Work out the finished part from the listing and answer in its coordinate system (mm). A direction names the side the tool comes from. Give positions to 0.01 mm unless a question says otherwise; leave off trailing zeros. Loops run counter-clockwise (first coordinate to the right, second up) from the corner with the lowest first, then second, coordinate; pieces in that order, holes last. Notation, with made-up numbers: M 48,-18.75 L 98,-18.75 A29 ccw 98,1.25 Z; hole C 17.5,-33 d2. An arc over 180 degrees is marked long. Use a Markdown table: item, result.
```python
from build123d import *

# Parameters (mm, degrees)
F1_DEPTH      = 10
F3_W          = 3
F3_H          = 10
F4_DEPTH      = 9.464
F5_W          = 7
F5_H          = 14
F5_W_2        = 3
F5_H_2        = 10
F6_DEPTH      = 3
F6_DEPTH_BACK = 1
F7_R          = 0.5


with BuildPart() as f1:
    # F0 (on Top) → F1 (new body)
    with BuildSketch(Plane.XY):
        Polygon((-13.856406, 0), (0, 0), (-3.464102, 6), align=None)
    extrude(amount=F1_DEPTH)

    # F3 (on offset) → F4 (join)
    with BuildSketch(Plane.YZ.offset(-3.4643)):
        with Locations((1.5, 5)):
            Rectangle(F3_W, F3_H)
    extrude(amount=F4_DEPTH)

    # F5 (on face) → F6 (join, two sides)
    with BuildSketch(Plane.YZ.offset(5.9997)) as f6_sk:
        with Locations((1.5, 5)):
            Rectangle(F5_W, F5_H)
        with Locations((1.5, 5)):
            Rectangle(F5_W_2, F5_H_2, mode=Mode.SUBTRACT)
    extrude(amount=F6_DEPTH)
    extrude(f6_sk.sketch, amount=-F6_DEPTH_BACK)

    # F7
    f7_edges = [f1.edges().sort_by_distance(p)[0] for p in [
        (-13.856406, 0, 5),
        (-3.464102, 6, 5),
    ]]
    fillet(f7_edges, radius=F7_R)


solid = f1.part
```
(1) A cutting plane is placed at D-D (y = 3.25). Write down the section's boundary in (x, z).
Entries:
| item | result |
|---|---|
| outline | M -8.23,0 L -1.88,0 L -1.88,10 L -8.23,10 Z; M 5,-2 L 9,-2 L 9,12 L 5,12 Z |
(2) Given P1, Ø3.5, axis at x = 3, z = 4, coming from the +Y side; P2, Ø8, axis at x = 4.5, z = 5.5, coming from the +Y side; P3, Ø3, axis at x = -2.5, y = 3.5, coming from the +Z side, each flat-ended and moving along its own axis, determine where each tip first touches the part or whether it passes through.
Entries:
| item | result |
|---|---|
| P1 | stops at y = 3 |
| P2 | stops at y = 5 |
| P3 | stops at z = 10 |
(3) A cutting plane is placed at A-A (y = 4.5). Write down the section's boundary in (x, z), and give its area (3 significant figures).
Entries:
| item | result |
|---|---|
| outline | M -6.06,0 L -2.6,0 L -2.6,10 L -6.06,10 Z; M 5,-2 L 9,-2 L 9,12 L 5,12 Z |
| area | 90.6 mm² |
(4) A cutting plane is placed at B-B (z = 8.75). Write down the section's boundary in (x, y), and give its area (3 significant figures).
Entries:
| item | result |
|---|---|
| outline | M -12.24,0.93 A0.5 ccw -11.99,0 L 5,0 L 5,-2 L 9,-2 L 9,0 L 6,0 L 6,3 L 9,3 L 9,5 L 5,5 L 5,3 L -1.73,3 L -3.21,5.57 A0.5 ccw -3.9,5.75 Z |
| area | 77.5 mm² |
(5) Consider probe 1 along Y at (x, z) = (7.5, 1); probe 2 along Z at (x, y) = (-4.75, 2.25); probe 3 along X at (y, z) = (-1.25, 0.25). Determine where each line is inside the solid, lowest interval first. Write a range as [from, to].
Entries:
| item | result |
|---|---|
| probe 1 | y = [-2, 0], [3, 5] |
| probe 2 | z = [0, 10] |
| probe 3 | x = [5, 9] |
(6) A cutting plane is placed at C-C (x = -1.5). Write down the section's boundary in (y, z).
Entries:
| item | result |
|---|---|
| outline | M 0,0 L 3,0 L 3,10 L 0,10 Z |
(7) Which of the six approach directions +Z, -Z, +X, -X, +Y, -Y give full straight-line access (tool end or side, diameter ignored) to faces 4 (the flat face through (-4, 0, 5)), 5 (the flat face through (7, 0, 5)), 6 (the flat face through (7, 5, 5)), 7 (the flat face through (2, 3, 5)), 8 (the flat face through (-4, 2, 0))?
Entries:
| item | result |
|---|---|
| face 4 | +Z, -Z, -X, -Y |
| face 5 | +X |
| face 6 | +Z, -Z, +X, +Y |
| face 7 | +Z, -Z, +Y |
| face 8 | -Z, -X, +Y, -Y |
(8) The mould has two halves that part along X. Classify faces 1 (the flat face through (-2.463, 4.266, 4.93)), 2 (the flat face through (-4, 2, 10)), 3 (the cylindrical face through (-12.47, 0.36, 5.07)): released by +X, released by -X, zero draft, split by the parting line, or undercut.
Entries:
| item | result |
|---|---|
| face 1 | undercut |
| face 2 | zero draft |
| face 3 | released by -X |
